from build123d import *

# Parameters (mm, degrees)
ESQUISSE1_W                  = 20
ESQUISSE1_H                  = 18
BOSS_EXTRU_1_DEPTH           = 17
ENL_V_MAT_EXTRU_1_DEPTH      = 32.827660926
ENL_V_MAT_EXTRU_1_DEPTH_BACK = 32.827660926
ESQUISSE4_W                  = 22.812140382
ESQUISSE4_H                  = 17.8
ENL_V_MAT_EXTRU_3_DEPTH      = 1
CONG_2_R                     = 40
ESQUISSE5_R                  = 2.1
ENL_V_MAT_EXTRU_4_DEPTH      = 29.861739379
CONG_3_R                     = 9
CHANFREIN1_SIZE              = 20.578216064
CHANFREIN1_SIZE_2            = 4
CONG_4_R                     = 6.05
ESQUISSE6_R                  = 1.1
ENL_V_MAT_EXTRU_5_DEPTH      = 252.816113418
ESQUISSE10_R                 = 1.9
ENL_V_MAT_EXTRU_6_DEPTH      = 7.5


# Some blends are built 0.0001 mm under size
with BuildPart() as part:
    # Esquisse1 → Boss.-Extru.1 (new body)
    with BuildSketch(Plane.XY):
        with Locations((10, 3)):
            Rectangle(ESQUISSE1_W, ESQUISSE1_H)
    extrude(amount=BOSS_EXTRU_1_DEPTH)

    # Esquisse2 → Enlèv. mat.-Extru.1 (cut, two sides: drawn at the far end of the back side and taken through both)
    with BuildSketch(Plane(origin=(0, 12, 0), x_dir=(1, 0, 0), z_dir=(0, 1, 0)).offset(-ENL_V_MAT_EXTRU_1_DEPTH_BACK)):
        Polygon((81.461522254, 11.626508335), (20.045630921, -0.0408989), (0, -3.849042594), (0, 0), (0, 62.514319158), (66.24104297, 168.553390377), (147.702565224, 117.665579555), align=None)
    extrude(amount=ENL_V_MAT_EXTRU_1_DEPTH + ENL_V_MAT_EXTRU_1_DEPTH_BACK, mode=Mode.SUBTRACT)

    # Esquisse4 → Enlèv. mat.-Extru.3 (cut)
    with BuildSketch(Plane(origin=(0.705746644, 0, 3.714969257), x_dir=(-0.9824291803850712, 0, 0.1866357562952965), z_dir=(-0.1866357562952965, 0, -0.9824291803850712))):
        with Locations((-8.233262334, 3)):
            Rectangle(ESQUISSE4_W, ESQUISSE4_H)
    extrude(amount=-ENL_V_MAT_EXTRU_3_DEPTH, mode=Mode.SUBTRACT)

    # Congé2
    # the kernel refuses this fillet: 40 mm, written as the material it adds along each edge
    with BuildSketch(Plane(origin=(41.830053891, 11.9, -3.079684565), x_dir=(0, -1, 0), z_dir=(-0.9824291803850712, 0, 0.1866357562952965))) as cong_2_piece_1_section:
        with BuildLine():
            CenterArc((8.888194417, -40), CONG_2_R, 90, 12.838568141)
            Line((0, -1), (0, 0))
            Line((0, 0), (8.888194417, 0))
        make_face()
    cong_2_piece_1 = extrude(amount=64.798673587, mode=Mode.PRIVATE)
    cong_2_piece_1 = split(cong_2_piece_1, bisect_by=Plane(origin=(20, 11.9, -3.079684565), z_dir=(-1, 0, 0)), keep=Keep.TOP, mode=Mode.PRIVATE)
    cong_2_piece_1 = split(cong_2_piece_1, bisect_by=Plane(origin=(0, 11.9, -3.079684565), z_dir=(1, 0, 0)), keep=Keep.TOP, mode=Mode.PRIVATE)
    add(cong_2_piece_1)
    with BuildSketch(Plane(origin=(-21.830053891, -5.9, 9.014064887), x_dir=(-0.1866357562952965, 0, -0.9824291803850712), z_dir=(0.9824291803850712, 0, -0.1866357562952965))) as cong_2_piece_2_section:
        with BuildLine():
            CenterArc((40, 8.888194417), CONG_2_R, 180, 12.838568141)
            Line((0, 8.888194417), (0, 0))
            Line((0, 0), (1, 0))
        make_face()
    cong_2_piece_2 = extrude(amount=64.798673587, mode=Mode.PRIVATE)
    cong_2_piece_2 = split(cong_2_piece_2, bisect_by=Plane(origin=(20, -5.9, 9.014064887), z_dir=(-1, 0, 0)), keep=Keep.TOP, mode=Mode.PRIVATE)
    cong_2_piece_2 = split(cong_2_piece_2, bisect_by=Plane(origin=(0, -5.9, 9.014064887), z_dir=(1, 0, 0)), keep=Keep.TOP, mode=Mode.PRIVATE)
    add(cong_2_piece_2)

    # Esquisse5 → Enlèv. mat.-Extru.4 (cut, through all)
    with BuildSketch(Plane.ZY):
        with Locations((10.5, 3)):
            Circle(ESQUISSE5_R)
    extrude(amount=-ENL_V_MAT_EXTRU_4_DEPTH, mode=Mode.SUBTRACT)

    # Congé3
    cong_3_edges = [part.edges().sort_by_distance(p)[0] for p in [
        (10, 12, 17),
        (10, -6, 17),
    ]]
    fillet(cong_3_edges, radius=CONG_3_R - 0.0001)  # a hair under: the kernel refuses the full size

    # Chanfrein1
    # the kernel refuses this chamfer: 20.578216064, 4 mm, written as the material it takes off along each edge
    with BuildSketch(Plane(origin=(20, -6, -53.417428004), x_dir=(-1, 0, 0), z_dir=(0, 0, 1))) as chanfrein1_piece_1:
        Polygon((CHANFREIN1_SIZE, 0), (0, -CHANFREIN1_SIZE_2), (0, 0), align=None)
    extrude(amount=61.417528004, mode=Mode.SUBTRACT)
    with BuildSketch(Plane(origin=(20, 2.9999, 8.0001), x_dir=(0, -1, 0), z_dir=(0, 0, -1))) as chanfrein1_piece_2:
        Polygon((8.9999, CHANFREIN1_SIZE), (8.9999 - CHANFREIN1_SIZE_2, 0), (8.9999, 0), align=None)
    revolve(axis=Axis((20, 2.9999, 8.0001), (-1, 0, 0)), revolution_arc=90, mode=Mode.SUBTRACT)
    with BuildSketch(Plane(origin=(20, 3.0001, 8.0001), x_dir=(0, 0, 1), z_dir=(0, -1, 0))) as chanfrein1_piece_3:
        Polygon((8.9999, CHANFREIN1_SIZE), (8.9999 - CHANFREIN1_SIZE_2, 0), (8.9999, 0), align=None)
    revolve(axis=Axis((20, 3.0001, 8.0001), (-1, 0, 0)), revolution_arc=90, mode=Mode.SUBTRACT)
    with BuildSketch(Plane(origin=(20, 12, -53.417428004), x_dir=(-1, 0, 0), z_dir=(0, 0, 1))) as chanfrein1_piece_4:
        Polygon((CHANFREIN1_SIZE, 0), (0, CHANFREIN1_SIZE_2), (0, 0), align=None)
    extrude(amount=61.417528004, mode=Mode.SUBTRACT)
    with BuildSketch(Plane(origin=(20, 2.9999, 17), x_dir=(-1, 0, 0), z_dir=(0, 1, 0))) as chanfrein1_piece_5:
        Polygon((CHANFREIN1_SIZE, 0), (0, -CHANFREIN1_SIZE_2), (0, 0), align=None)
    extrude(amount=0.0002, mode=Mode.SUBTRACT)

    # Congé4
    # the kernel refuses this fillet: 6.05 mm, written as the material it takes off along each edge
    with BuildSketch(Plane(origin=(20, -2, -11.718464458), x_dir=(-0.9816271834478701, -0.1908089953754837, 0), z_dir=(0, 0, 1))) as cong_4_piece_1:
        with BuildLine():
            CenterArc((CONG_4_R * 0.824336385818, -CONG_4_R), CONG_4_R, 90, 79)
            Line((-CONG_4_R * 0.157290797629, -CONG_4_R * 0.809191004625), (0, 0))
            Line((0, 0), (CONG_4_R * 0.824336385818, 0))
        make_face()
    extrude(amount=19.718564458, mode=Mode.SUBTRACT)
    with BuildSketch(Plane(origin=(20, 2.9999, 8.0001), x_dir=(0, -1, 0), z_dir=(0, 0, -1))) as cong_4_piece_2:
        with BuildLine():
            CenterArc((4.9999 - CONG_4_R * 0.824336385818, CONG_4_R), CONG_4_R, 270, 79)
            Line((4.9999 - CONG_4_R * 0.824336385818, 0), (4.9999, 0))
            Line((4.9999, 0), (4.9999 + CONG_4_R * 0.157290797629, CONG_4_R * 0.809191004625))
        make_face()
    revolve(axis=Axis((20, 2.9999, 8.0001), (-1, 0, 0)), revolution_arc=90, mode=Mode.SUBTRACT)
    with BuildSketch(Plane(origin=(20, 3.0001, 8.0001), x_dir=(0, 0, 1), z_dir=(0, -1, 0))) as cong_4_piece_3:
        with BuildLine():
            CenterArc((4.9999 - CONG_4_R * 0.824336385818, CONG_4_R), CONG_4_R, 270, 79)
            Line((4.9999 - CONG_4_R * 0.824336385818, 0), (4.9999, 0))
            Line((4.9999, 0), (4.9999 + CONG_4_R * 0.157290797629, CONG_4_R * 0.809191004625))
        make_face()
    revolve(axis=Axis((20, 3.0001, 8.0001), (-1, 0, 0)), revolution_arc=90, mode=Mode.SUBTRACT)
    with BuildSketch(Plane(origin=(20, 8, -11.718464458), x_dir=(-0.9816271834478701, 0.1908089953754837, 0), z_dir=(0, 0, 1))) as cong_4_piece_4:
        with BuildLine():
            CenterArc((CONG_4_R * 0.824336385818, CONG_4_R), CONG_4_R, 191, 79)
            Line((-CONG_4_R * 0.157290797629, CONG_4_R * 0.809191004625), (0, 0))
            Line((0, 0), (CONG_4_R * 0.824336385818, 0))
        make_face()
    extrude(amount=19.718564458, mode=Mode.SUBTRACT)
    with BuildSketch(Plane(origin=(20, 2.9999, 13), x_dir=(-0.9816271834478701, 0, 0.1908089953754837), z_dir=(0, 1, 0))) as cong_4_piece_5:
        with BuildLine():
            CenterArc((CONG_4_R * 0.824336385818, -CONG_4_R), CONG_4_R, 90, 79)
            Line((-CONG_4_R * 0.157290797629, -CONG_4_R * 0.809191004625), (0, 0))
            Line((0, 0), (CONG_4_R * 0.824336385818, 0))
        make_face()
    extrude(amount=0.0002, mode=Mode.SUBTRACT)

    # Esquisse6 → Enlèv. mat.-Extru.5 (cut, through all)
    with BuildSketch(Plane(origin=(247.804103642, 0, -26.276800017), x_dir=(-0.9824291803850712, 0, 0.1866357562952965), z_dir=(-0.1866357562952965, 0, -0.9824291803850712))):
        with Locations(Location((244, 7.9, 0), (0, 0, 180))):
            Circle(ESQUISSE6_R)
        with Locations(Location((244, -1.9, 0), (0, 0, 180))):
            Circle(ESQUISSE6_R)
    extrude(amount=ENL_V_MAT_EXTRU_5_DEPTH, mode=Mode.SUBTRACT)

    # Esquisse10 → Enlèv. mat.-Extru.6 (cut)
    with BuildSketch(Plane(origin=(3.813717133, 0, 20.074968868), x_dir=(-0.9824291803850712, 0, 0.1866357562952965), z_dir=(-0.1866357562952965, 0, -0.9824291803850712))):
        with Locations((-4.4, 7.9)):
            Circle(ESQUISSE10_R)
        with Locations((-4.4, -1.9)):
            Circle(ESQUISSE10_R)
    extrude(amount=ENL_V_MAT_EXTRU_6_DEPTH, mode=Mode.SUBTRACT)


solid = part.part
Source: CAD feature listing. Evaluate the final solid. Frame: model axes, mm. A direction names the side the tool comes from. Round coordinates to 2 decimals unless told otherwise and drop trailing zeros.
Q1. Section A-A, the plane z = 10.5. State how many separate pieces and enclosed holes the cut face has, plus the area to 3 significant figures.
Q2. Ray query, line 1 (Y direction, x = 4.25, z = 4.25); line 2 (Z direction, x = 16.25, y = 1.5); line 3 (Y direction, x = 14.75, z = 10.5). Return the intervals inside material, ascending.
Q3. First-contact query: P1, Ø6, axis at x = 17, y = 1, coming from the +Z side; P2, Ø4, axis at x = 5.5, y = 8, coming from the +Z side; P3, Ø4, axis at x = 4.5, y = 0.5, coming from the -Z side. Flat tips, straight axial feed; report the tip coordinate or a pass-through.
Q4. Mould query, pull axis Z, two halves, no side actions, for faces 1 (the face through (9.83, -0.43, 2.85)), 2 (the face through (9.336, -2.056, 12.946)), 3 (the face through (6, 9, 8)). Classes: pulls with the +Z half, pulls with the -Z half, needs draft (parallel to the pull), parting line crosses it, or undercut.
Q5. Access query for faces 4 (the face through (7.89, 6.43, 3.22)), 5 (the face through (7.592, -0.975, 11.723)), 6 (the face through (9.85, 3.09, 8.4)). Directions: +Z, -Z, +X, -X, +Y, -Y. A direction counts if a zero-diameter tool reaches every point of the face in a straight line with its end or side. Return the directions, or none.
Solutions:
1. separate pieces: 2
1. enclosed holes: 2
1. area: 157 mm2
2. line 1: y = -5.06 to -2.41, -1.39 to 7.39, 8.41 to 11.06
2. line 2: z = 1.75 to 9.03, 11.97 to 13.4
2. line 3: y = -2.48 to 0.9, 5.1 to 8.48
3. P1: stops at z = 14.07
3. P2: stops at z = 15.32
3. P3: stops at z = 3.53
4. face 1: pulls with the -Z half
4. face 2: pulls with the +Z half
4. face 3: undercut
5. face 4: -Z, -X
5. face 5: none
5. face 6: +X, -X
